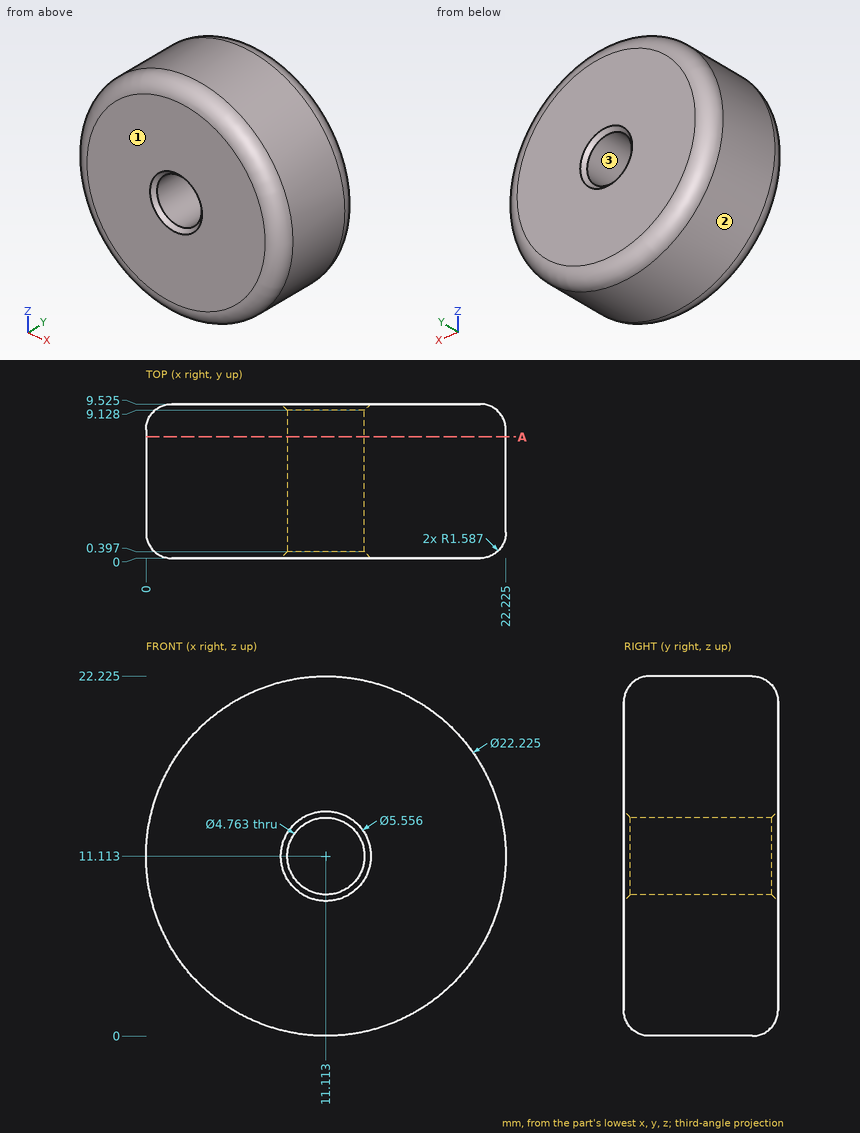
Answer from the drawing. Dimensions are ordinates in mm from the lowest x, y and z of the part. Give positions to 0.01 mm unless a question says otherwise; leave off trailing zeros. Write each loop counter-clockwise with the first axis right and the second up, starting at its lowest first coordinate (ties: lowest second). Pieces come first, ordered by that corner, then holes. Notation, with made-up numbers: (71, 68) - (87, 68) arc R22 cw to (87, 86) - close; hole circle Ø4 at (77, 84). An arc over 180 degrees is marked (long way). One line per item, written item: value. Start each with the question number.
1. Given pin 1 (1.5 mm diameter, centred on x = 3, z = 12.5, fed in from -Y); pin 2 (4 mm diameter, centred on x = 4, y = 5.5, fed in from -Z) (1 decimal); pin 3 (2 mm diameter, centred on x = 13, y = 6.5, fed in from -Z) (1 decimal); pin 4 (1.5 mm diameter, centred on x = 7, y = 1.5, fed in from +Z), each flat-ended and moving along its own axis, determine where each tip first touches the part or whether it passes through.
2. Consider probe 1 along X at (y, z) = (7.25, 11) (1 decimal); probe 2 along X at (y, z) = (6, 9.75) (1 decimal); probe 3 along Z at (x, y) = (10.5, 6) (1 decimal). Determine where each line is inside the solid, lowest interval first.
3. Find section A-A (y = 7.5). Write down the section's boundary in (x, z) (1 decimal).
4. For a pull along Z with two mould halves and no side action, classify the marked faces 1, 2 and 3 as +Z half, -Z half, draft (parallel to the pull), parting line (faces both ways), or undercut.
Geometry results:
1. pin 1: y = 0
1. pin 2: z = 1.2
1. pin 3: z = 0
1. pin 4: z = 21.7
2. probe 1: 0 to 8.7, 13.5 to 22.2
2. probe 2: 0.1 to 9.2, 13.1 to 22.1
2. probe 3: 0 to 8.8, 13.4 to 22.2
3. outline: circle Ø22.2 at (11.1, 11.1); hole circle Ø4.8 at (11.1, 11.1)
4. face 1: draft
4. face 2: parting line
4. face 3: undercut
